Verification items for this drawing (mm, ordinates from the low corner). A direction names the side the tool comes from. Coordinates: 2 decimals unless noted, no trailing zeros. Loops run counter-clockwise (first coordinate to the right, second up) from the corner with the lowest first, then second, coordinate; pieces in that order, holes last. Notation, with made-up numbers: M -20.75,23.25 L 35.25,23.25 A26 cw 35.25,53.25 Z; hole C -8,4.25 d8. An arc over 180 degrees is marked long. Return JSON: item names as keys, results as strings.
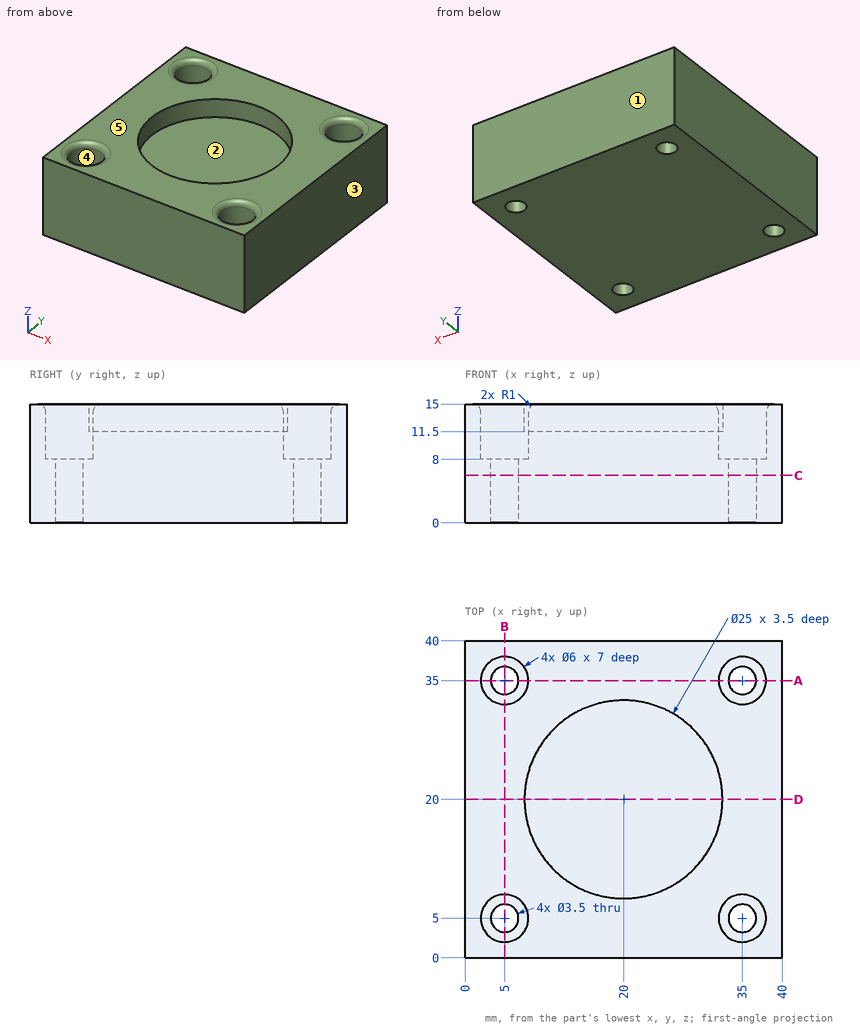
1) Draft check along X on the marked faces 1, 2 and 3. Enter one of: +X half, -X half, draft (parallel to the pull), parting line (faces both ways), or undercut.
Answers:
{"face 1": "draft", "face 2": "undercut", "face 3": "+X half"}
2) Go/stop test with flat-tipped pins: pin 1 Ø5 at (x, y) = (35, 35) entering from +Z; pin 2 Ø3 at (x, z) = (29, 3) entering from -Y; pin 3 Ø3 at (x, y) = (5, 5) entering from +Z; pin 4 Ø4 at (x, y) = (25.5, 20.5) entering from +Z. Record where each tip stops, or that it passes through.
Answers:
{"pin 1": "z = 8", "pin 2": "y = 0", "pin 3": "through", "pin 4": "z = 11.5"}
3) Scan lines: line 1 along Y through (x, z) = (5, 12.2); line 2 along Y through (x, z) = (35, 3.5); line 3 along Y through (x, z) = (20, 13.8). Record each from-to range of solid material in increasing order. Write a range as [from, to].
Answers:
{"line 1": "[0, 2], [8, 32], [38, 40]", "line 2": "[0, 3.25], [6.75, 33.25], [36.75, 40]", "line 3": "[0, 7.5], [32.5, 40]"}
4) Set-up check for the marked faces 4 and 5: record each of +Z, -Z, +X, -X, +Y, -Y from which the full face is reachable in a straight line by a thin tool's end or side.
Answers:
{"face 4": "+Z", "face 5": "+Z, +X, -X, +Y, -Y"}
5) Section check A-A on y = 35. Record the cut outline in (x, z).
Answers:
{"outline": "M 0,0 L 3.25,0 L 3.25,8 L 2,8 L 2,14 A1 ccw 1,15 L 0,15 Z; M 6.75,0 L 33.25,0 L 33.25,8 L 32,8 L 32,14 A1 ccw 31,15 L 9,15 A1 ccw 8,14 L 8,8 L 6.75,8 Z; M 36.75,0 L 40,0 L 40,15 L 39,15 A1 ccw 38,14 L 38,8 L 36.75,8 Z"}
6) Section check C-C on z = 6. Record the cut outline in (x, y).
Answers:
{"outline": "M 0,0 L 40,0 L 40,40 L 0,40 Z; hole C 5,5 d3.5; hole C 5,35 d3.5; hole C 35,5 d3.5; hole C 35,35 d3.5"}
7) Section check D-D on y = 20. Record the cut outline in (x, z).
Answers:
{"outline": "M 0,0 L 40,0 L 40,15 L 32.5,15 L 32.5,11.5 L 7.5,11.5 L 7.5,15 L 0,15 Z"}
